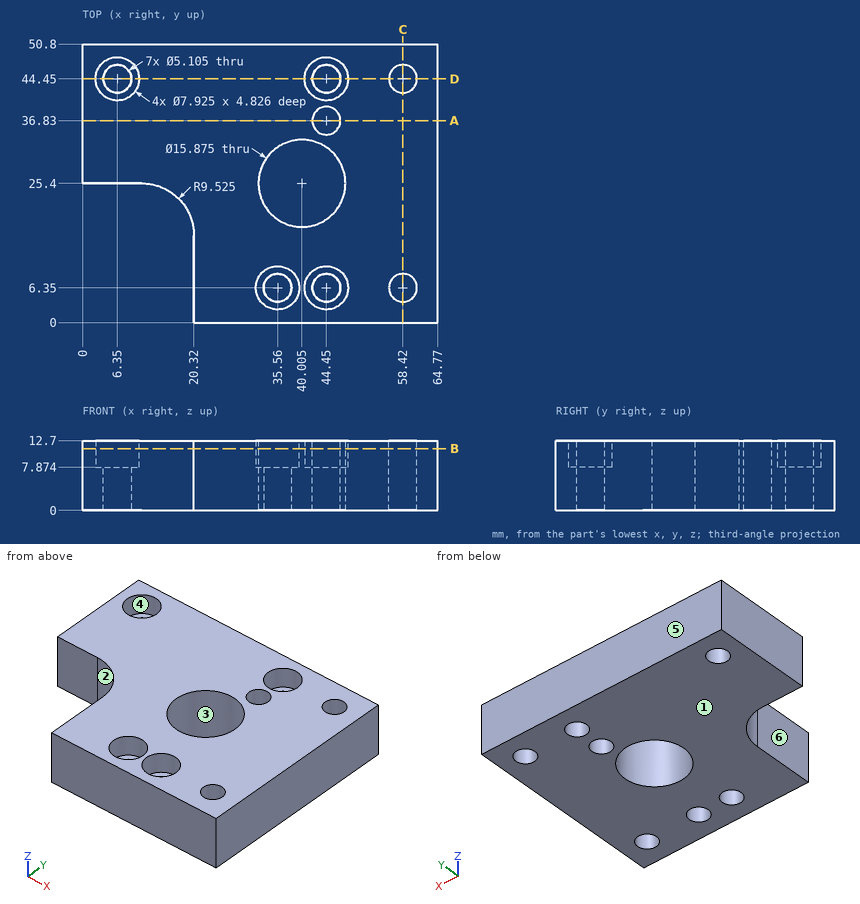
Geometry check sheet. Reference: drawing and pictorial views, mm from the part's lowest x, y, z. A direction names the side the tool comes from. Round coordinates to 2 decimals unless told otherwise and drop trailing zeros. Order: outer loops, then holes, each group sorted by start corner. A loop starts at its lowest first (then second) coordinate and runs counter-clockwise, first axis right, second up. Notation, with made-up numbers: M 9,18 L 25,18 A13 ccw 25,26 Z; hole C 81,89 d10. An arc over 180 degrees is marked long. Answer as CSV lines item,"result".
1) Sectioned sample at B-B on z = 11.25. Give the number of separate pieces and of enclosed holes in the cut face, and give its area (3 significant figures).
Entries:
separate pieces,"1"
enclosed holes,"8"
area,"2,340 mm2"
2) Sectioned sample at D-D on y = 44.45. Record the cut outline in (x, z), and give its area (3 significant figures).
Entries:
outline,"M 0,0 L 3.8,0 L 3.8,7.87 L 2.39,7.87 L 2.39,12.7 L 0,12.7 Z; M 8.9,0 L 41.9,0 L 41.9,7.87 L 40.49,7.87 L 40.49,12.7 L 10.31,12.7 L 10.31,7.87 L 8.9,7.87 Z; M 47,0 L 55.87,0 L 55.87,12.7 L 48.41,12.7 L 48.41,7.87 L 47,7.87 Z; M 60.97,0 L 64.77,0 L 64.77,12.7 L 60.97,12.7 Z"
area,"601 mm2"
3) Tool access check on the marked faces 4, 5 and 6. Record the directions out of +Z, -Z, +X, -X, +Y, -Y that give a thin tool (end or side, any length) a straight path to the whole face; none if there is none.
Entries:
face 4,"+Z"
face 5,"+Z, -Z, +X, -X, +Y"
face 6,"+Z, -Z, -X, -Y"
4) Sectioned sample at A-A on y = 36.83. Record the cut outline in (x, z).
Entries:
outline,"M 0,0 L 41.9,0 L 41.9,12.7 L 0,12.7 Z; M 47,0 L 64.77,0 L 64.77,12.7 L 47,12.7 Z"
5) Sectioned sample at C-C on x = 58.42. Record the cut outline in (y, z).
Entries:
outline,"M 0,0 L 3.8,0 L 3.8,12.7 L 0,12.7 Z; M 8.9,0 L 41.9,0 L 41.9,12.7 L 8.9,12.7 Z; M 47,0 L 50.8,0 L 50.8,12.7 L 47,12.7 Z"
6) Thickness scan on probe 1 along Y at (x, z) = (58.42, 9.25); probe 2 along X at (y, z) = (6.5, 3); probe 3 along Y at (x, z) = (44.45, 11.05) (1 decimal). Record the ranges inside material, lowest first. Write a range as [from, to].
Entries:
probe 1,"[0, 3.8], [8.9, 41.9], [47, 50.8]"
probe 2,"[20.32, 33.01], [38.11, 41.9], [47, 55.87], [60.97, 64.77]"
probe 3,"[0, 2.4], [10.3, 18.8], [32, 34.3], [39.4, 40.5], [48.4, 50.8]"
7) Gauge pin test, flat ends, axial feed: pin 1 Ø8.5 at (x, y) = (43.5, 45.5) entering from +Z; pin 2 Ø2 at (x, y) = (14.5, 22.5) entering from -Z; pin 3 Ø5.5 at (x, z) = (7.5, 4) entering from -Y. Record the tip position at first contact, or that the pin passes through.
Entries:
pin 1,"z = 12.7"
pin 2,"through"
pin 3,"y = 25.4"
8) Mould release check, pull along X, two halves, no side actions. Record for the marked faces 1, 2 and 3: +X half, -X half, draft (parallel to the pull), parting line (faces both ways), or undercut.
Entries:
face 1,"draft"
face 2,"-X half"
face 3,"undercut"
